The figure shows three views and two pictorial views of one solid part (mm, origin at its lowest corner). Answer the questions. Round coordinates to 2 decimals unless told otherwise and drop trailing zeros. Loops run counter-clockwise (first coordinate to the right, second up) from the corner with the lowest first, then second, coordinate; pieces in that order, holes last. Notation, with made-up numbers: (32.25, -16) -> (74.25, -16) arc R25 cw to (74.25, 14) -> close; hole circle Ø1 at (58.5, 33). An arc over 180 degrees is marked (long way). Put each result on its own line as item: value.
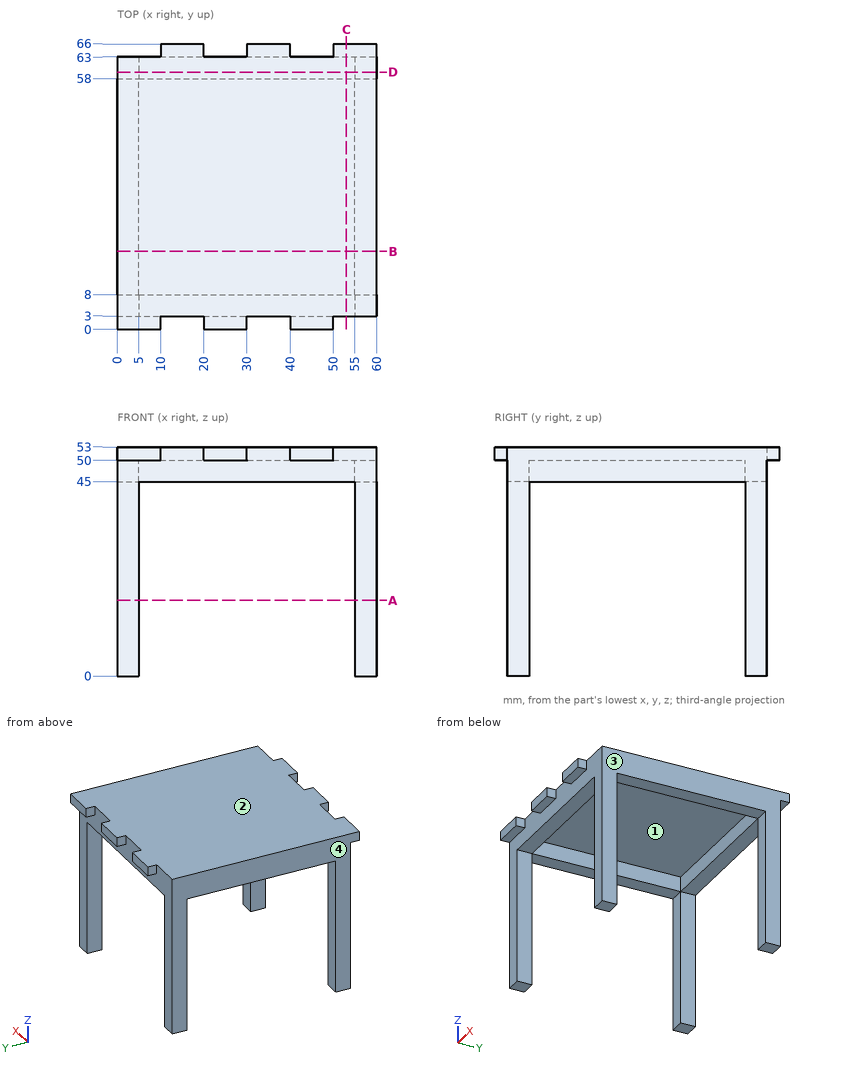
Item 1: The part is cut by section B-B (y = 18). Determine the outline of the cut face in (x, z).
Derived:
outline: (0, 45) -> (5, 45) -> (5, 50) -> (55, 50) -> (55, 45) -> (60, 45) -> (60, 53) -> (0, 53) -> close
Item 2: Find the intervals of material crossed by line 1 along Y through (x, z) = (26, 48); line 2 along X through (y, z) = (53, 46.5); line 3 along Z through (x, y) = (5.5, 34), in increasing order.
Derived:
line 1: y = 3 to 8, 58 to 63
line 2: x = 0 to 5, 55 to 60
line 3: z = 50 to 53
Item 3: The part is cut by section D-D (y = 59.5). Determine the outline of the cut face in (x, z).
Derived:
outline: (0, 0) -> (5, 0) -> (5, 45) -> (55, 45) -> (55, 0) -> (60, 0) -> (60, 53) -> (0, 53) -> close
Item 4: The part is cut by section A-A (z = 17.5). Determine the outline of the cut face in (x, y).
Derived:
outline: (0, 3) -> (5, 3) -> (5, 8) -> (0, 8) -> close; (0, 58) -> (5, 58) -> (5, 63) -> (0, 63) -> close; (55, 3) -> (60, 3) -> (60, 8) -> (55, 8) -> close; (55, 58) -> (60, 58) -> (60, 63) -> (55, 63) -> close
Item 5: Flat-ended cylindrical pins translate along their axes: pin 1 Ø2.5 at (x, y) = (29.5, 5.5) entering from -Z; pin 2 Ø1.5 at (y, z) = (1, 52) entering from +X; pin 3 Ø0.9 at (x, y) = (36.5, 65) entering from -Z. Find the tip coordinate at first contact, or state that the pin passes through.
Derived:
pin 1: stops at z = 45
pin 2: stops at x = 50
pin 3: stops at z = 50
Item 6: For a pull along X with two mould halves and no side action, classify the marked faces 1, 2, 3 and 4 as pulls with the +X half, pulls with the -X half, needs draft (parallel to the pull), parting line crosses it, or undercut.
Derived:
face 1: undercut
face 2: needs draft
face 3: pulls with the +X half
face 4: pulls with the -X half
Item 7: The part is cut by section C-C (x = 53). Determine the outline of the cut face in (y, z).
Derived:
outline: (3, 45) -> (8, 45) -> (8, 50) -> (58, 50) -> (58, 45) -> (63, 45) -> (63, 50) -> (66, 50) -> (66, 53) -> (3, 53) -> close
